from build123d import *

# Parameters (mm, degrees)
SKETCH1_R           = 3.575
BOSS_EXTRUDE1_DEPTH = 3
THREAD1_PITCH       = 1


with BuildPart() as part:
    # Sketch1 → Boss-Extrude1 (new body)
    with BuildSketch(Plane(origin=(0, 0, 0), x_dir=(1, 0, 0), z_dir=(0, 1, 0))):
        Polygon((7, 0), (3.5, 6.062177826), (-3.5, 6.062177826), (-7, 0), (-3.5, -6.062177826), (3.5, -6.062177826), align=None)
        with Locations(Location((0, 0, 0), (0, 0, 270))):
            Circle(SKETCH1_R, mode=Mode.SUBTRACT)
    extrude(amount=BOSS_EXTRUDE1_DEPTH)

    # Thread1: the profile of Thread Profile1 profile screwed along a right-hand helix of 3 turns, 8 arcs to a turn; built about Z, then put on its axis
    thread1_z = Axis((0, 0, 0), (0, 0, 1))
    thread1_corners = [(3.5747, 0, -0.000173205), (4.116265875, 0, 0.312499999), (4.116265875, 0, 0.437499999), (3.5747, 0, 0.750173202)]
    with BuildLine(mode=Mode.PRIVATE) as thread1_profile:
        Line(thread1_corners[0], thread1_corners[1])
        Line(thread1_corners[1], thread1_corners[2])
        Line(thread1_corners[2], thread1_corners[3])
        Line(thread1_corners[3], thread1_corners[0])
    thread1_cap = Face(thread1_profile.wire())
    thread1_turn_angles = [0, 22.5, 45, 67.5, 90, 112.5, 135, 157.5, 180, 202.5, 225, 247.5, 270, 292.5, 315, 337.5, 360]
    thread1_turn_weights = [1, 0.9238795325112867, 1, 0.9238795325112867, 1, 0.9238795325112867, 1, 0.9238795325112867, 1, 0.9238795325112867, 1, 0.9238795325112867, 1, 0.9238795325112867, 1, 0.9238795325112867, 1]
    thread1_turn_rails = [Edge.make_bspline([Vector(p[0], p[1], 0).rotate(thread1_z, thread1_turn_angles[k]) / thread1_turn_weights[k] + Vector(0, 0, p[2] + THREAD1_PITCH * thread1_turn_angles[k] / 360) for k in range(17)], [0, 0, 0, 1, 1, 2, 2, 3, 3, 4, 4, 5, 5, 6, 6, 7, 7, 8, 8, 8], 2, thread1_turn_weights) for p in thread1_corners]
    thread1_turn_sides = [Face.make_surface_from_curves(thread1_turn_rails[p[0]], thread1_turn_rails[p[1]]) for p in [(0, 1), (1, 2), (2, 3), (3, 0)]]
    thread1 = Plane(origin=(0, 3, 0), x_dir=(-1, 0, 0), z_dir=(0, -1, 0)) * Solid(Shell([*[p.moved(Location((0, 0, THREAD1_PITCH * i))) for i in range(3) for p in thread1_turn_sides], thread1_cap, thread1_cap.rotate(thread1_z, 1080).moved(Location((0, 0, THREAD1_PITCH * 1080 / 360)))]))
    add(thread1, mode=Mode.SUBTRACT)


solid = part.part
Build history of the part. All positions in model axes, mm. Coordinates: 2 decimals unless noted, no trailing zeros. Order: outer loops, then holes, each group sorted by start corner. A loop starts at its lowest first (then second) coordinate and runs counter-clockwise, first axis right, second up. Notation, with made-up numbers: M -24.5,-5 L 25.5,-5 A18 cw 25.5,30 Z; hole C -1,33 d3. An arc over 180 degrees is marked long. One line per question, with ' | ' between items. Start each with the question number.
Q1. Saw through at A-A (z = 5). List the corners of the cut face in (x, y), then the cut area to 3 significant figures.
Q2. Two-plate mould, pull along X, no slides. Class faces 1 (the face through (-5.274, 1.479, 2.989)), 2 (the face through (5.226, 1.479, 3.074)), 3 (the face through (0, 1, 6.062)): +X half, -X half, draft (parallel to the pull), parting line (faces both ways), or undercut.
Q3. Probe L1, parallel to Y at x = -4, z = -0.75; L2, parallel to Z at x = 0, y = 1.85 (3 decimals); L3, parallel to Z at x = 0, y = 2.65 (3 decimals). List the from-to ranges inside material, lowest first. Write a range as from..to.
Q4. Flat gauge pins, fed straight in: pin 1 Ø0.6 at (x, y) = (-4, 2.5) entering from -Z; pin 2 Ø1.5 at (x, y) = (4.5, 0.5) entering from -Z. Where does each tip first touch, or does it go through?
Q5. Saw through at B-B (x = 6.25). List the corners of the cut face in (y, z), then the cut area to 3 significant figures.
Check values:
1) outline: M -4.11,0 L 4.11,0 L 4.11,3 L -4.11,3 Z | area: 24.7 mm2
2) face 1: -X half | face 2: +X half | face 3: draft
3) L1: y = 0..0.51, 0.69..1.51, 1.69..2.51, 2.69..3 | L2: z = -6.062..-3.575, 4.116..6.062 | L3: z = -6.062..-3.748, 3.575..6.062
4) pin 1: stops at z = -5.72 | pin 2: stops at z = -5.63
5) outline: M 0,-1.3 L 3,-1.3 L 3,1.3 L 0,1.3 Z | area: 7.79 mm2
